```python
from build123d import *

# Parameters (mm, degrees)
SKETCH1_W            = 82.55
SKETCH1_H            = 95.25
BOSS_EXTRUDE1_DEPTH  = 3.175
SKETCH2_W            = 3.175
SKETCH2_H            = 4.7625
CUT_EXTRUDE1_DEPTH   = 64.101876953
LPATTERN1_COUNT      = 2
LPATTERN1_PITCH      = 76.2
LPATTERN1_COUNT_DIR2 = 2
LPATTERN1_PITCH_DIR2 = 73.025


with BuildPart() as part:
    # Sketch1 → Boss-Extrude1 (new body)
    with BuildSketch(Plane(origin=(0, 0, 0), x_dir=(1, 0, 0), z_dir=(0, 1, 0))):
        Rectangle(SKETCH1_W, SKETCH1_H)
    extrude(amount=BOSS_EXTRUDE1_DEPTH)

    # Sketch2 → Cut-Extrude1 (cut, through all)
    with BuildSketch(Plane(origin=(0, 3.175, 0), x_dir=(1, 0, 0), z_dir=(0, 1, 0))):
        with Locations((-36.5125, 42.06875)):
            Rectangle(SKETCH2_W, SKETCH2_H)
        with Locations((-36.5125, 34.13125)):
            Rectangle(SKETCH2_W, SKETCH2_H)
    cut_extrude1 = extrude(amount=-CUT_EXTRUDE1_DEPTH, mode=Mode.SUBTRACT)

    # LPattern1: Cut-Extrude1 2 × 2
    with Locations(*[(j * LPATTERN1_PITCH_DIR2, 0, i * LPATTERN1_PITCH) for i in range(LPATTERN1_COUNT) for j in range(LPATTERN1_COUNT_DIR2) if (i, j) != (0, 0)]):
        add(cut_extrude1, mode=Mode.SUBTRACT)


solid = part.part
```
Model file for the job. Use its own axes, mm. Give positions to 0.01 mm unless a question says otherwise; leave off trailing zeros. Use one line per item in the form item = value.
Item 1: Two-plate mould, pull along Z, no slides. Class faces 1 (the flat face through (-1, 3.175, -1)), 2 (the flat face through (-1, 2, -47.625)), 3 (the flat face through (34.925, 2, 34)): released by +Z, released by -Z, zero draft, split by the parting line, or undercut.
Filled in:
face_1 = zero draft
face_2 = released by -Z
face_3 = undercut
Item 2: Drill centre line: L1, parallel to X at y = 1.95, z = -40.5 (3 decimals). Where is it in solid material? Low to high.
Filled in:
L1 = -41.275 to -38.1, -34.925 to 34.925, 38.1 to 41.275
Item 3: Slice it at A-A on y = 1.6. Give the number of separate pieces and of enclosed holes in the cut face, and give its area (3 significant figures).
Filled in:
separate_pieces = 1
enclosed_holes = 8
area = 7,740 mm^2
